Design review of the part shown in the three views and the two pictorial views. Dimensions are in mm from the part's minimum x, y and z. A direction names the side the tool comes from. Give positions to 0.01 mm unless a question says otherwise; leave off trailing zeros. Order: outer loops, then holes, each group sorted by start corner. A loop starts at its lowest first (then second) coordinate and runs counter-clockwise, first axis right, second up.
Item 1: For probe 1 along X at (y, z) = (25.5, 2.75); probe 2 along X at (y, z) = (47, 7.25); probe 3 along Z at (x, y) = (47.5, 47.5), list the stretches that pass through material, from the lowest coordinate up.
Item 2: Consider section D-D (z = 25). Give the boundary of the cut face in (x, y).
Item 3: Machinability: for the marked faces 1, 2 and 3, which of the approach directions +Z, -Z, +X, -X, +Y, -Y give a long, thin tool a straight path to every point of the face, cutting with its end or side? Answer none if there is none.
Item 4: Consider section A-A (z = 4). Give the boundary of the cut face in (x, y), plus the area to 3 significant figures.
Item 5: The part is to be moulded in two halves that separate along X. For the marked faces 4, 5, 6 and 7, say which applies: released by +X, released by -X, zero draft, split by the parting line, or undercut.
Item 6: For P1, Ø3, axis at y = 41, z = 23.5, coming from the +X side; P2, Ø9.5, axis at x = 70.5, y = 31, coming from the +Z side; P3, Ø5, axis at y = 22.5, z = 4.5, coming from the -X side, all flat-tipped, find the tip position at first contact; note any pin that passes through.
Item 7: Consider section C-C (x = 17.5). Give the boundary of the cut face in (y, z), plus the area to 3 significant figures.
Item 8: Consider section B-B (y = 34). Give the boundary of the cut face in (x, z) (1 decimal), plus the area to 3 significant figures.
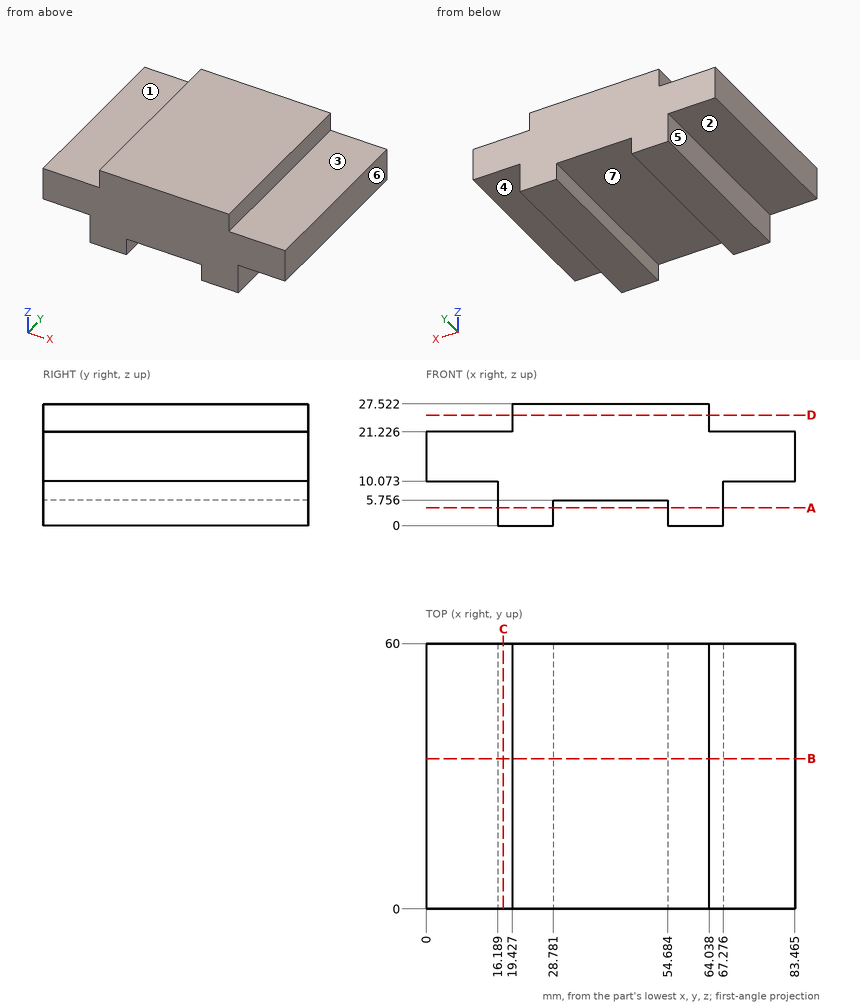
Resolved:
1. probe 1: x = 16.19 to 28.78, 54.68 to 67.28
1. probe 2: x = 16.19 to 67.28
1. probe 3: z = 5.76 to 27.52
2. outline: (19.43, 0) - (64.04, 0) - (64.04, 60) - (19.43, 60) - close
3. face 1: +Z, -X, +Y, -Y
3. face 2: -Z, -X, +Y, -Y
3. face 3: +Z, +X, +Y, -Y
4. outline: (16.19, 0) - (28.78, 0) - (28.78, 60) - (16.19, 60) - close; (54.68, 0) - (67.28, 0) - (67.28, 60) - (54.68, 60) - close
4. area: 1,510 mm2
5. face 4: zero draft
5. face 5: released by -X
5. face 6: released by +X
5. face 7: undercut
6. P1: stops at x = 64.04
6. P2: stops at z = 21.23
6. P3: stops at x = 16.19
7. outline: (0, 0) - (60, 0) - (60, 21.23) - (0, 21.23) - close
7. area: 1,270 mm2
8. outline: (0, 10.1) - (16.2, 10.1) - (16.2, 0) - (28.8, 0) - (28.8, 5.8) - (54.7, 5.8) - (54.7, 0) - (67.3, 0) - (67.3, 10.1) - (83.5, 10.1) - (83.5, 21.2) - (64, 21.2) - (64, 27.5) - (19.4, 27.5) - (19.4, 21.2) - (0, 21.2) - close
8. area: 1,580 mm2
